from build123d import *

# Parameters (mm, degrees)
F1_DEPTH = 1
F3_DEPTH = 1.5
F5_DEPTH = 2.5


with BuildPart() as f1:
    # F0 (on Front) → F1 (new body)
    with BuildSketch(Plane.XZ):
        with BuildLine():
            ThreePointArc((0, 2), (0.5857864376, 0.5857864376), (2, 0))
            Line((2, 0), (40, 0))
            ThreePointArc((40, 0), (41.4142135624, 0.5857864376), (42, 2))
            Line((42, 2), (42, 25))
            Line((42, 25), (0, 25))
            Line((0, 25), (0, 2))
        make_face()
    extrude(amount=F1_DEPTH)

    # F2 (on face) → F3 (join)
    with BuildSketch(Plane.XZ.offset(1)):
        with BuildLine():
            Line((39.75, 25), (2.25, 25))
            Line((2.25, 25), (2.25, 2))
            ThreePointArc((2.25, 2), (2.8357864376, 0.5857864376), (4.25, 0))
            Line((4.25, 0), (37.75, 0))
            ThreePointArc((37.75, 0), (39.1642135624, 0.5857864376), (39.75, 2))
            Line((39.75, 2), (39.75, 25))
        make_face()
    extrude(amount=F3_DEPTH)

    # F4 (on face) → F5 (cut, through all)
    with BuildSketch(Plane.XZ.offset(2.5)):
        with BuildLine():
            Line((35, 8.5), (7, 8.5))
            ThreePointArc((7, 8.5), (4.5, 6), (7, 3.5))
            Line((7, 3.5), (35, 3.5))
            ThreePointArc((35, 3.5), (37.5, 6), (35, 8.5))
        make_face()
    extrude(amount=-F5_DEPTH, mode=Mode.SUBTRACT)


solid = f1.part
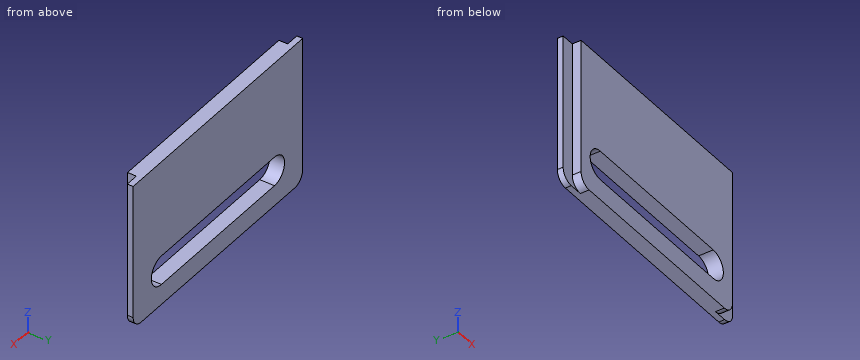
Build history of the part. All positions in model axes, mm. Give positions to 0.01 mm unless a question says otherwise; leave off trailing zeros. Order: outer loops, then holes, each group sorted by start corner. A loop starts at its lowest first (then second) coordinate and runs counter-clockwise, first axis right, second up. Notation, with made-up numbers: M 4,-33.75 L 29,-33.75 A20 cw 29,-25.75 Z; hole C 32,29.25 d11. An arc over 180 degrees is marked long. Put each result on its own line as item: value.
Item 1: Cut at C-C on x = 29. Write the cut outline in (y, z), then the cut area to 3 significant figures.
Results are:
outline: M -2.5,0 L 0,0 L 0,3.5 L -2.5,3.5 Z; M -2.5,8.5 L 0,8.5 L 0,25 L -2.5,25 Z
area: 50.0 mm2
Item 2: Cut at A-A on z = 8. Write the cut outline in (x, y).
Results are:
outline: M 0,-1 L 2.25,-1 L 2.25,-2.5 L 5.5,-2.5 L 5.5,0 L 0,0 Z; M 36.5,-2.5 L 39.75,-2.5 L 39.75,-1 L 42,-1 L 42,0 L 36.5,0 Z
Item 3: Drop a flat-ended pin along its axis: pin 1 Ø1.2 at (y, z) = (-2, 17.5) entering from -X. Give the stop position or say it passes through.
Results are:
pin 1: x = 2.25
Item 4: Cut at B-B on y = -1.65. Write the cut outline in (x, z), then the cut area to 3 significant figures.
Results are:
outline: M 2.25,2 A2 ccw 4.25,0 L 37.75,0 A2 ccw 39.75,2 L 39.75,25 L 2.25,25 Z; hole M 7,3.5 L 35,3.5 A2.5 ccw 35,8.5 L 7,8.5 A2.5 ccw Z
area: 776 mm2
Item 5: Wall check: probe 1 along Z at (x, y) = (35, -0.8); probe 2 along X at (y, z) = (-2, 9); probe 3 along Z at (x, y) = (5.5, -1.45). Give the ranges that are in metal, low to high.
Results are:
probe 1: 0 to 3.5, 8.5 to 25
probe 2: 2.25 to 39.75
probe 3: 0 to 4, 8 to 25
Item 6: Cut at D-D on z = 15. Write the cut outline in (x, y).
Results are:
outline: M 0,-1 L 2.25,-1 L 2.25,-2.5 L 39.75,-2.5 L 39.75,-1 L 42,-1 L 42,0 L 0,0 Z
